from build123d import *

# Parameters (mm, degrees)
SKETCH1_W               = 80
SKETCH1_H               = 60
SKETCH1_W_2             = 75.6
SKETCH1_H_2             = 55.6
BOSS_EXTRUDE1_DEPTH     = 40
CHAMFER1_SIZE           = 18
SKETCH2_W               = 60
SKETCH2_H               = 20
BOSS_EXTRUDE2_DEPTH     = 1.8
SKETCH5_W               = 80
SKETCH5_H               = 50
SKETCH5_W_2             = 75.6
SKETCH5_H_2             = 45.6
BOSS_EXTRUDE3_DEPTH     = 40
SKETCH6_W               = 80
SKETCH6_H               = 10
CUT_EXTRUDE3_DEPTH      = 40
SKETCH7_R               = 1.6
SKETCH7_R_2             = 6.4
SKETCH7_R_3             = 3
CUT_EXTRUDE4_DEPTH      = 40
CUT_EXTRUDE5_DEPTH      = 101.761302096
CUT_EXTRUDE5_DEPTH_BACK = 40
SKETCH3_R               = 1.5
SKETCH4_R               = 3.25
SKETCH4_R_2             = 6.125
CUT_EXTRUDE6_DEPTH      = 103.46950766
SKETCH10_W              = 80
SKETCH10_H              = 40
BOSS_EXTRUDE4_DEPTH     = 1
SKETCH12_W              = 15
SKETCH12_H              = 5
CUT_EXTRUDE10_DEPTH     = 103.46950766
SKETCH13_W              = 5
SKETCH13_H              = 15
CUT_EXTRUDE11_DEPTH     = 10
CUT_EXTRUDE12_DEPTH     = 75.560311158
BOSS_EXTRUDE5_START     = -1.2
BOSS_EXTRUDE5_DEPTH     = 15
BOSS_EXTRUDE8_DEPTH     = 2
CHAMFER2_SIZE           = 3
CHAMFER3_SIZE           = 3
CUT_EXTRUDE15_START     = -1.2
CUT_EXTRUDE15_DEPTH     = 2.2
CUT_EXTRUDE16_START     = -2.2
SKETCH26_R              = 3.75
CUT_EXTRUDE16_DEPTH     = 2.2
BOSS_EXTRUDE9_START     = -25
SKETCH27_W              = 2
SKETCH27_H              = 8
BOSS_EXTRUDE9_DEPTH     = 15
FILLET1_R               = 1
SKETCH28_W              = 8
SKETCH28_H              = 2
BOSS_EXTRUDE10_DEPTH    = 40
FILLET2_R               = 1
CUT_EXTRUDE17_DEPTH     = 101.761302096


with BuildPart() as part:
    # Sketch1 → Boss-Extrude1 (new body)
    # profile 1 of 2: a face of its own
    with BuildSketch(Plane.XY):
        Polygon((-30, 50), (-30, 30), (30, 30), (30, 50), (27.8, 50), (27.8, 47.8), (27.8, 32.2), (-27.8, 32.2), (-27.8, 47.8), (-27.8, 50), align=None)
    # profile 2 of 2: a face of its own
    with BuildSketch(Plane.XY):
        Rectangle(SKETCH1_W, SKETCH1_H)
        Rectangle(SKETCH1_W_2, SKETCH1_H_2, mode=Mode.SUBTRACT)
    extrude(amount=BOSS_EXTRUDE1_DEPTH)

    # Chamfer1
    # the kernel refuses this chamfer: 18 mm, written as the material it takes off along each edge
    with BuildSketch(Plane(origin=(76.290293783, 50, 40), x_dir=(0, -0.9996219169112966, 0.02749587661058639), z_dir=(-1, 0, 0)), Plane(origin=(18.490293783, 50, 40), x_dir=(0, -0.9996219169112966, 0.02749587661058639), z_dir=(-1, 0, 0))) as chamfer1_piece_1:
        Polygon((CHAMFER1_SIZE * 0.999621916911, -CHAMFER1_SIZE * 0.0274958766106), (-CHAMFER1_SIZE * 0.0274958766106, -CHAMFER1_SIZE * 0.999621916911), (0, 0), align=None)
    extrude(amount=94.780587567, mode=Mode.SUBTRACT)

    # Sketch2 → Boss-Extrude2 (add)
    with BuildSketch(Plane(origin=(0, 0, 0), x_dir=(-1, 0, 0), z_dir=(0, 0, -1))):
        with Locations((0, 40)):
            Rectangle(SKETCH2_W, SKETCH2_H)
    extrude(amount=-BOSS_EXTRUDE2_DEPTH)

    # Sketch5 → Boss-Extrude3 (add)
    with BuildSketch(Plane.XY.offset(40)):
        with Locations((0, 5)):
            Rectangle(SKETCH5_W, SKETCH5_H)
        with Locations((0, 5)):
            Rectangle(SKETCH5_W_2, SKETCH5_H_2, mode=Mode.SUBTRACT)
    extrude(amount=-BOSS_EXTRUDE3_DEPTH)

    # Sketch6 → Cut-Extrude3 (cut)
    with BuildSketch(Plane.XY.offset(40)):
        with Locations((0, -25)):
            Rectangle(SKETCH6_W, SKETCH6_H)
    extrude(amount=-CUT_EXTRUDE3_DEPTH, mode=Mode.SUBTRACT)

    # Sketch7 → Cut-Extrude4 (cut)
    with BuildSketch(Plane.XZ.offset(-27.8)):
        with Locations((0, 2.3)):
            Circle(SKETCH7_R)
        with Locations((0, 21.75)):
            Circle(SKETCH7_R_2)
        with Locations((0, 15.45)):
            Circle(SKETCH7_R_3)
        with Locations((0, 30.3)):
            Circle(SKETCH7_R)
    extrude(amount=-CUT_EXTRUDE4_DEPTH, mode=Mode.SUBTRACT)

    # Sketch3 → Cut-Extrude5 (cut, two sides: drawn at the far end of the back side and taken through both)
    with BuildSketch(Plane.ZY.offset(-37.8).offset(-CUT_EXTRUDE5_DEPTH_BACK)):
        with Locations((34, 15)):
            Circle(SKETCH3_R)
        with Locations((5.8, 15)):
            Circle(SKETCH3_R)
    extrude(amount=CUT_EXTRUDE5_DEPTH + CUT_EXTRUDE5_DEPTH_BACK, mode=Mode.SUBTRACT)

    # Sketch4 → Cut-Extrude6 (cut, through all)
    with BuildSketch(Plane(origin=(40, 0, 0), x_dir=(0, 0, -1), z_dir=(1, 0, 0))):
        with Locations((-18.95, 15)):
            Circle(SKETCH4_R)
        with Locations((-25.25, 15)):
            Circle(SKETCH4_R_2)
    extrude(amount=-CUT_EXTRUDE6_DEPTH, mode=Mode.SUBTRACT)

    # Sketch10 → Boss-Extrude4 (add)
    with BuildSketch(Plane(origin=(0, -17.8, 0), x_dir=(1, 0, 0), z_dir=(0, 1, 0))):
        with Locations((0, -20)):
            Rectangle(SKETCH10_W, SKETCH10_H)
    extrude(amount=BOSS_EXTRUDE4_DEPTH)

    # Sketch12 → Cut-Extrude10 (cut, through all)
    with BuildSketch(Plane.ZY.offset(40)):
        with Locations((20, -2.5)):
            Rectangle(SKETCH12_W, SKETCH12_H)
    extrude(amount=-CUT_EXTRUDE10_DEPTH, mode=Mode.SUBTRACT)

    # Sketch13 → Cut-Extrude11 (cut)
    with BuildSketch(Plane.XZ.offset(20)):
        with Locations((-34.5, 12.5)):
            Rectangle(SKETCH13_W, SKETCH13_H)
        with Locations((34.5, 12.5)):
            Rectangle(SKETCH13_W, SKETCH13_H)
    extrude(amount=-CUT_EXTRUDE11_DEPTH, mode=Mode.SUBTRACT)

    # Sketch14 → Cut-Extrude12 (cut, through all)
    with BuildSketch(Plane.XY.offset(1.8)):
        Polygon((-27.8, 50), (-24.469302189, 38.708703588), (-14.659934208, 32.2), (14.659934208, 32), (24.505699212, 38.608703588), (27.8, 50), align=None)
    extrude(amount=-CUT_EXTRUDE12_DEPTH, mode=Mode.SUBTRACT)

    # Sketch15 → Boss-Extrude5 (add)
    with BuildSketch(Plane.XY.offset(1.8).offset(BOSS_EXTRUDE5_START)):
        Polygon((27.8, 50), (24.505699212, 38.608703588), (14.957897791, 32.2), (-14.659934208, 32.2), (-24.469302189, 38.708703588), (-27.8, 50), (-29.718283002, 50), (-29.718283002, 49.434146376), (-26.181631315, 37.44465205), (-15.765700543, 30.53348243), (16.07253082, 30.539399744), (26.224741306, 37.353796576), (29.721271707, 49.444378702), (29.721271707, 50), align=None)
    extrude(amount=-BOSS_EXTRUDE5_DEPTH)

    # Sketch22 → Boss-Extrude8 (add)
    with BuildSketch(Plane(origin=(0, 0, -14.4), x_dir=(-1, 0, 0), z_dir=(0, 0, -1))):
        Polygon((-26.224741306, 37.353796576), (-16.07253082, 30.539399744), (15.765700543, 30.53348243), (26.181631315, 37.44465205), (29.718283002, 49.434146376), (29.718283002, 50), (27.8, 50), (24.469302189, 38.708703588), (14.659934208, 32.2), (-14.957897791, 32.2), (-24.505699212, 38.608703588), (-27.8, 50), (-29.721271707, 50), (-29.721271707, 49.444378702), align=None)
        Polygon((-27.8, 50), (27.8, 50), (24.469302189, 38.708703588), (14.659934208, 32.2), (-14.957897791, 32.2), (-24.505699212, 38.608703588), align=None)
    extrude(amount=BOSS_EXTRUDE8_DEPTH)

    # Chamfer2
    chamfer2_edges = [part.edges().sort_by_distance(p)[0] for p in [
        (37.8, 27.8, 20),
        (-37.8, 27.8, 20),
    ]]
    chamfer(chamfer2_edges, length=CHAMFER2_SIZE)

    # Chamfer3
    chamfer3_edges = [part.edges().sort_by_distance(p)[0] for p in [
        (40, 30, 20),
        (-40, 30, 20),
    ]]
    chamfer(chamfer3_edges, length=CHAMFER3_SIZE)

    # Sketch25 → Cut-Extrude15 (cut)
    with BuildSketch(Plane.XZ.offset(20).offset(CUT_EXTRUDE15_START)):
        with BuildLine():
            Line((-3.634615385, 20.923076923), (-1.75, 36))
            ThreePointArc((-1.75, 36), (0, 37.75), (1.75, 36))
            Line((1.75, 36), (3.634615385, 20.923076923))
            ThreePointArc((3.634615385, 20.923076923), (0, 16.25), (-3.634615385, 20.923076923))
        make_face()
    extrude(amount=-CUT_EXTRUDE15_DEPTH, mode=Mode.SUBTRACT)

    # Sketch26 → Cut-Extrude16 (cut)
    with BuildSketch(Plane(origin=(0, -18.8, 0), x_dir=(1, 0, 0), z_dir=(0, 1, 0)).offset(CUT_EXTRUDE16_START)):
        with Locations(Location((0, -20, 0), (0, 0, 90))):
            Circle(SKETCH26_R)
    extrude(amount=CUT_EXTRUDE16_DEPTH, mode=Mode.SUBTRACT)

    # Sketch27 → Boss-Extrude9 (add)
    with BuildSketch(Plane.XY.offset(40).offset(BOSS_EXTRUDE9_START)):
        with Locations((-1.7, -12.8)):
            Rectangle(SKETCH27_W, SKETCH27_H)
    extrude(amount=-BOSS_EXTRUDE9_DEPTH)

    # Fillet1
    fillet1_edges = [part.edges().sort_by_distance(p)[0] for p in [
        (-0.7, -16.8, 7.5),
        (-2.7, -16.8, 7.5),
    ]]
    fillet(fillet1_edges, radius=FILLET1_R)

    # Sketch28 → Boss-Extrude10 (add)
    with BuildSketch(Plane.XY.offset(40)):
        with Locations((33.8, 5.7)):
            Rectangle(SKETCH28_W, SKETCH28_H)
    extrude(amount=-BOSS_EXTRUDE10_DEPTH)

    # Fillet2
    fillet2_edges = [part.edges().sort_by_distance(p)[0] for p in [
        (37.8, 6.7, 20),
        (37.8, 4.7, 20),
    ]]
    fillet(fillet2_edges, radius=FILLET2_R)

    # Sketch29 → Cut-Extrude17 (cut, through all)
    with BuildSketch(Plane(origin=(-37.8, 0, 0), x_dir=(0, 0, -1), z_dir=(1, 0, 0))):
        with BuildLine():
            Line((-34.4, -11.8), (-27.8, -11.8))
            ThreePointArc((-27.8, -11.8), (-27.092893219, -12.092893219), (-26.8, -12.8))
            Line((-26.8, -12.8), (-26.8, -14.8))
            ThreePointArc((-26.8, -14.8), (-27.092893219, -15.507106781), (-27.8, -15.8))
            Line((-27.8, -15.8), (-34.4, -15.8))
            ThreePointArc((-34.4, -15.8), (-35.107106781, -15.507106781), (-35.4, -14.8))
            Line((-35.4, -14.8), (-35.4, -12.8))
            ThreePointArc((-35.4, -12.8), (-35.107106781, -12.092893219), (-34.4, -11.8))
        make_face()
        with BuildLine():
            Line((-21.8, -11.8), (-15.2, -11.8))
            ThreePointArc((-15.2, -11.8), (-14.492893219, -12.092893219), (-14.2, -12.8))
            Line((-14.2, -12.8), (-14.2, -14.8))
            ThreePointArc((-14.2, -14.8), (-14.492893219, -15.507106781), (-15.2, -15.8))
            Line((-15.2, -15.8), (-21.8, -15.8))
            ThreePointArc((-21.8, -15.8), (-22.507106781, -15.507106781), (-22.8, -14.8))
            Line((-22.8, -14.8), (-22.8, -12.8))
            ThreePointArc((-22.8, -12.8), (-22.507106781, -12.092893219), (-21.8, -11.8))
        make_face()
    extrude(amount=-CUT_EXTRUDE17_DEPTH, mode=Mode.SUBTRACT)


solid = part.part
Verification items for the finished model (mm, model axes). A direction names the side the tool comes from. Coordinates: 2 decimals unless noted, no trailing zeros. Order: outer loops, then holes, each group sorted by start corner. A loop starts at its lowest first (then second) coordinate and runs counter-clockwise, first axis right, second up. Notation, with made-up numbers: M -29.75,68 L -2.75,68 A7 ccw -2.75,72 Z; hole C 43,60.25 d6. An arc over 180 degrees is marked long. One line per item, written item: value. Start each with the question number.
Item 1: Sectioned sample at B-B (x = -31). Enter the section's corners in (y, z).
Item 2: Sectioned sample at A-A (y = 2.5). Enter the section's corners in (x, z), then the cut area to 3 significant figures.
Item 3: Access from +Z, -Z, +X, -X, +Y, -Y to the whole of each face (thin tool, end or side, straight path). Record for faces 1 (the flat face through (0, 32.2, -7)), 2 (the flat face through (39, -5, 20)), 3 (the flat face through (-39, -15.8, 18)), 4 (the cylindrical face through (-0.04, -17.81, 37.75)), 5 (the flat face through (37.8, 16, 15)).
Item 4: Gauge pin test, flat ends, axial feed: pin 1 (9 mm diameter, centred on x = -3.5, y = 37.5, fed in from +Z); pin 2 (5 mm diameter, centred on y = 15, z = 18.95, fed in from +X); pin 3 (6.5 mm diameter, centred on x = 20.5, y = 38, fed in from +Z); pin 4 (1.8 mm diameter, centred on x = -38.5, z = 32, fed in from +Y). Record the tip position at first contact, or that the pin passes through.
Item 5: Scan lines: probe 1 along Z at (x, y) = (0, 28.7); probe 2 along X at (y, z) = (38, 4); probe 3 along Y at (x, z) = (-39, 18). Record each from-to range of solid material in increasing order.
Item 6: Mould release check, pull along X, two halves, no side actions. Record for faces 6 (the flat face through (-0.7, -12, 8)), 7 (the flat face through (-34, 30, 20)), 8 (the flat face through (-38, 29, 20)): released by +X, released by -X, zero draft, split by the parting line, or undercut.
Conclusion:
1. outline: M -20,0 L -16.8,0 L -16.8,40 L -20,40 Z; M 27.8,0 L 30,0 L 30,40 L 27.8,40 Z
2. outline: M -40,0 L -37.8,0 L -37.8,40 L -40,40 Z; M 37.8,0 L 40,0 L 40,40 L 37.8,40 Z
2. area: 176 mm^2
3. face 1: +Z, +Y
3. face 2: +X, -X
3. face 3: -X
3. face 4: none
3. face 5: +Z, -Z
4. pin 1: stops at z = -14.4
4. pin 2: passes through
4. pin 3: stops at z = 1.8
4. pin 4: stops at y = 29.4
5. probe 1: z = 0 to 0.7, 3.9 to 12.45, 28.15 to 28.7, 31.9 to 40
5. probe 2: x = -30 to -27.8, 27.8 to 30
5. probe 3: y = -20 to -15.8, -11.8 to -5, 0 to 11.89, 18.11 to 28
6. face 6: undercut
6. face 7: zero draft
6. face 8: released by -X
